Geometry check sheet. Reference: the model listing, model coordinates, mm. A direction names the side the tool comes from. Round coordinates to 2 decimals unless told otherwise and drop trailing zeros. Order: outer loops, then holes, each group sorted by start corner. A loop starts at its lowest first (then second) coordinate and runs counter-clockwise, first axis right, second up. Notation, with made-up numbers: (-40, -37) - (15, -37) arc R26 cw to (15, -1) - close; hole circle Ø11 at (-22.75, 64.5). An arc over 180 degrees is marked (long way). One line per question, with ' | ' between items. Start each with the question number.
Q1. Sectioned sample at A-A, the plane z = 8.75. Enter the section's corners in (x, y), then the cut area to 3 significant figures.
Q2. Mould release check, pull along Y, two halves, no side actions. Record for faces 3 (the face through (161, 109, 10)), 4 (the face through (161, 6, 9)), 5 (the face through (157, 55, 0)): +Y half, -Y half, draft (parallel to the pull), parting line (faces both ways), or undercut.
Q3. Sectioned sample at B-B, the plane x = 49.5. Enter the section's corners in (y, z), then the cut area to 3 significant figures.
Q4. Sectioned sample at C-C, the plane y = 60.5. Enter the section's corners in (x, z).
Q5. Material ranges on line 1 along X through (y, z) = (92, 7.25); line 2 along Y through (x, z) = (188, 10.25); line 3 along Y through (x, z) = (149.5, 14.25), recorded low to high.
Q6. Tool access check on faces 1 (the face through (318, 54, 10)), 2 (the face through (157, 103, 9)). Record the directions out of +Z, -Z, +X, -X, +Y, -Y that give a thin tool (end or side, any length) a straight path to the whole face; none if there is none.
Q7. Gauge pin test, flat end, axial feed: P1, Ø1, axis at x = 101, y = 29.5, coming from the +Z side. Record the tip position at first contact, or that the pin passes through.
Solid Edge part; units mm, degrees
sketch "Sketch1" plane through (0, 0, 0) normal (0, 0, 1) x (1, 0, 0)
  line L0 (0, 0) -> (318, 0)
  line L1 (318, 0) -> (318, 109)
  line L2 (318, 109) -> (0, 109)
  line L3 (0, 109) -> (0, 0)
extrude "Protrusion1" add sketch "Sketch1" along normal blind 21
sketch "Sketch2" plane through (159, 54.5, 21) normal (0, 0, 1) x (1, 0, 0)
  line L0 (-153, 48.5) -> (153, 48.5)
  line L1 (153, 48.5) -> (153, -48.5)
  line L2 (153, -48.5) -> (-153, -48.5)
  line L3 (-153, -48.5) -> (-153, 48.5)
extrude "ExtrudedCutout_1" cut sketch "Sketch2" against normal blind 17
sketch "Sketch3" plane through (159, 54.5, 21) normal (0, 0, 1) x (1, 0, 0)
  line L0 (-155, 50.5) -> (155, 50.5)
  line L1 (155, 50.5) -> (155, -50.5)
  line L2 (155, -50.5) -> (-155, -50.5)
  line L3 (-155, -50.5) -> (-155, 50.5)
extrude "Cutout1" cut sketch "Sketch3" against normal blind 7.6
Determined:
1) outline: (0, 0) - (318, 0) - (318, 109) - (0, 109) - close; hole (6, 6) - (312, 6) - (312, 103) - (6, 103) - close | area: 4,980 mm2
2) face 3: +Y half | face 4: undercut | face 5: draft
3) outline: (0, 0) - (109, 0) - (109, 21) - (105, 21) - (105, 13.4) - (103, 13.4) - (103, 4) - (6, 4) - (6, 13.4) - (4, 13.4) - (4, 21) - (0, 21) - close | area: 610 mm2
4) outline: (0, 0) - (318, 0) - (318, 21) - (314, 21) - (314, 13.4) - (312, 13.4) - (312, 4) - (6, 4) - (6, 13.4) - (4, 13.4) - (4, 21) - (0, 21) - close
5) line 1: x = 0 to 6, 312 to 318 | line 2: y = 0 to 6, 103 to 109 | line 3: y = 0 to 4, 105 to 109
6) face 1: +Z, -Z, +X, +Y, -Y | face 2: +Z
7) P1: stops at z = 4
